```python
from build123d import *

# Parameters (mm, degrees)
EXTRUDE_1_DEPTH            = 50
HOLE_WIZARD_M6_D           = 6.6
HOLE_WIZARD_M6_CSINK_D     = 12.6
HOLE_WIZARD_M6_CSINK_ANGLE = 90
HOLE_WIZARD_M4_D           = 4.5
HOLE_WIZARD_M4_CSINK_D     = 9.4
HOLE_WIZARD_M4_CSINK_ANGLE = 90
CHAMFER_1_SIZE             = 0.5


with BuildPart() as part:
    # Эскиз1 → Бобышка-Вытянуть1 (new body)
    with BuildSketch(Plane.XY):
        Polygon((0, 0), (5.3, 0), (5.3, 1.2), (17, 1.2), (17, 11.2), (-17, 11.2), (-17, 1.2), (-5.3, 1.2), (-5.3, 0), align=None)
    extrude(amount=-EXTRUDE_1_DEPTH)

    # Винт M6 (through all)
    with Locations(Plane(origin=(0, 11.2, 0), x_dir=(1, 0, 0), z_dir=(0, 1, 0))):
        with Locations((0, 25)):
            CounterSinkHole(HOLE_WIZARD_M6_D / 2, HOLE_WIZARD_M6_CSINK_D / 2, counter_sink_angle=HOLE_WIZARD_M6_CSINK_ANGLE)

    # Винт M4 (through all)
    with Locations(Plane(origin=(0, 1.2, 0), x_dir=(-1, 0, 0), z_dir=(0, -1, 0))):
        with Locations((12, 5), (-12, 5), (12, 45), (-12, 45)):
            CounterSinkHole(HOLE_WIZARD_M4_D / 2, HOLE_WIZARD_M4_CSINK_D / 2, counter_sink_angle=HOLE_WIZARD_M4_CSINK_ANGLE)

    # Фаска1
    chamfer_1_edges = [part.edges().sort_by_distance(p)[0] for p in [
        (-5.3, 0, -25),
        (5.3, 0, -25),
    ]]
    chamfer(chamfer_1_edges, length=CHAMFER_1_SIZE)


solid = part.part
```
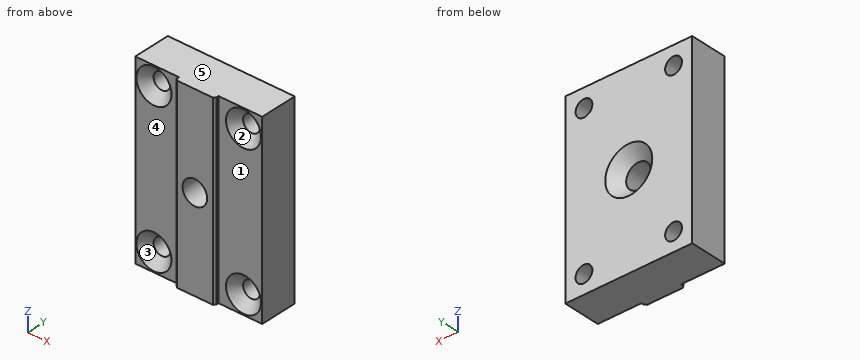
Design review of the part built by this model. Coordinates are the model's own, in mm. Face numbers are marked on the shaded views. A direction names the side the tool comes from. Give positions to 0.01 mm unless a question says otherwise; leave off trailing zeros. Order: outer loops, then holes, each group sorted by start corner. A loop starts at its lowest first (then second) coordinate and runs counter-clockwise, first axis right, second up. Notation, with made-up numbers: (71.25, -3.75) - (95.25, -3.75) arc R18 cw to (95.25, 13.25) - close; hole circle Ø8 at (-8.5, -32.75). An arc over 180 degrees is marked (long way). Use a Markdown table: item, result. Add a question column.
(1) Clearance check with flat-ended pins moving along their axes: P1, Ø2, axis at x = 6, z = -34.5, coming from the -Y side; P2, Ø6, axis at x = -12, z = -45, coming from the -Y side; P3, Ø9.5, axis at x = -12, z = -14.5, coming from the -Y side; P4, Ø3.5, axis at x = 12, z = -45, coming from the +Y side. State where each tip first meets the part, or that it passes through.
(2) Add section D-D on y = 6. Give the boundary of the cut face in (x, z), then the cut area to 3 significant figures.
(3) Add section C-C on z = -25. Give the boundary of the cut face in (x, y).
(4) Wall thickness on probe 1 along Z at (x, y) = (-12, 7.25); probe 2 along X at (y, z) = (6, -45); probe 3 along Z at (x, y) = (-15, 2.5): over which ranges is each line inside the solid? List them lowest first. Write a range as [from, to].
(5) Add section B-B on x = 0. Give the boundary of the cut face in (y, z).
(6) Mouldability with a two-part tool opening along Z and no side actions: class the marked faces 3, 4 and 5 as +Z half, -Z half, draft (parallel to the pull), parting line (faces both ways), or undercut.
(7) Add section A-A on z = -5. Give the boundary of the cut face in (x, y), then the cut area to 3 significant figures.
(8) Machinability: for the marked faces 1 and 2, which of the approach directions +Z, -Z, +X, -X, +Y, -Y give a long, thin tool a straight path to every point of the face, cutting with its end or side? Answer none if there is none.
Report:
| question | item | result |
|---|---|---|
| 1 | P1 | stops at y = 0.2 |
| 1 | P2 | stops at y = 2.9 |
| 1 | P3 | stops at y = 1.2 |
| 1 | P4 | passes through |
| 2 | outline | (-17, -50) - (17, -50) - (17, 0) - (-17, 0) - close; hole circle Ø4.5 at (-12, -45); hole circle Ø4.5 at (-12, -5); hole circle Ø6.6 at (0, -25); hole circle Ø4.5 at (12, -45); hole circle Ø4.5 at (12, -5) |
| 2 | area | 1,600 mm² |
| 3 | outline | (-17, 1.2) - (-5.3, 1.2) - (-5.3, 0.5) - (-4.8, 0) - (-3.3, 0) - (-3.3, 8.2) - (-6.3, 11.2) - (-17, 11.2) - close; (3.3, 0) - (4.8, 0) - (5.3, 0.5) - (5.3, 1.2) - (17, 1.2) - (17, 11.2) - (6.3, 11.2) - (3.3, 8.2) - close |
| 4 | probe 1 | z = [-50, -47.25], [-42.75, -7.25], [-2.75, 0] |
| 4 | probe 2 | x = [-17, -14.25], [-9.75, 9.75], [14.25, 17] |
| 4 | probe 3 | z = [-50, -46.6], [-43.4, -6.6], [-3.4, 0] |
| 5 | outline | (0, -50) - (11.2, -50) - (11.2, -31.3) - (8.2, -28.3) - (0, -28.3) - close; (0, -21.7) - (8.2, -21.7) - (11.2, -18.7) - (11.2, 0) - (0, 0) - close |
| 6 | face 3 | undercut |
| 6 | face 4 | draft |
| 6 | face 5 | +Z half |
| 7 | outline | (-17, 1.2) - (-16.7, 1.2) - (-14.25, 3.65) - (-14.25, 11.2) - (-17, 11.2) - close; (-9.75, 3.65) - (-7.3, 1.2) - (-5.3, 1.2) - (-5.3, 0.5) - (-4.8, 0) - (4.8, 0) - (5.3, 0.5) - (5.3, 1.2) - (7.3, 1.2) - (9.75, 3.65) - (9.75, 11.2) - (-9.75, 11.2) - close; (14.25, 3.65) - (16.7, 1.2) - (17, 1.2) - (17, 11.2) - (14.25, 11.2) - close |
| 7 | area | 250 mm² |
| 8 | face 1 | +Z, -Z, +X, -Y |
| 8 | face 2 | -Y |
